Here's how the part is built. I have some questions about the finished solid (model axes, mm). A direction names the side the tool comes from. Coordinates: 2 decimals unless noted, no trailing zeros. Write each loop counter-clockwise with the first axis right and the second up, starting at its lowest first coordinate (ties: lowest second). Pieces come first, ordered by that corner, then holes. Notation, with made-up numbers: (34.5, 66.25) -> (54.5, 66.25) arc R23 ccw to (54.5, 98.25) -> close; hole circle Ø7 at (54, -7). An arc over 180 degrees is marked (long way). Answer in a Markdown table with one row per item. Add a question column.
from build123d import *

# Parameters (mm, degrees)
SKETCH2_R           = 19.05
SKETCH2_R_2         = 6.688770164
SKETCH2_R_3         = 2.328803663
BOSS_EXTRUDE1_DEPTH = 6.35
SKETCH3_R           = 10.424468921
BOSS_EXTRUDE2_DEPTH = 11.176
FILLET1_R           = 2.54


with BuildPart() as part:
    # Sketch2 → Boss-Extrude1 (new body)
    with BuildSketch(Plane(origin=(0, 0, 0), x_dir=(1, 0, 0), z_dir=(0, 1, 0))):
        with Locations(Location((0, 0, 0), (0, 0, 270))):
            Circle(SKETCH2_R)
        with Locations(Location((0, 0, 0), (0, 0, 270))):
            Circle(SKETCH2_R_2, mode=Mode.SUBTRACT)
        with Locations(Location((0, 13.4441798, 0), (0, 0, 270))):
            Circle(SKETCH2_R_3, mode=Mode.SUBTRACT)
        with Locations(Location((13.4441798, 0, 0), (0, 0, 270))):
            Circle(SKETCH2_R_3, mode=Mode.SUBTRACT)
        with Locations(Location((0, -13.4441798, 0), (0, 0, 270))):
            Circle(SKETCH2_R_3, mode=Mode.SUBTRACT)
        with Locations(Location((-13.4441798, 0, 0), (0, 0, 270))):
            Circle(SKETCH2_R_3, mode=Mode.SUBTRACT)
    extrude(amount=BOSS_EXTRUDE1_DEPTH)

    # Sketch3 → Boss-Extrude2 (add)
    with BuildSketch(Plane(origin=(0, 6.35, 0), x_dir=(1, 0, 0), z_dir=(0, 1, 0))):
        with Locations(Location((0, 0, 0), (0, 0, 270))):
            Circle(SKETCH3_R)
    extrude(amount=BOSS_EXTRUDE2_DEPTH)

    # Fillet1
    fillet1_edges = [part.edges().sort_by_distance(p)[0] for p in [
        (0, 17.526, -10.424468921),
    ]]
    fillet(fillet1_edges, radius=FILLET1_R)


with BuildPart() as body_2:
    # Sketch5 → Revolve1 (revolve)
    with BuildSketch(Plane(origin=(0, 17.526, 0), x_dir=(1, 0, 0), z_dir=(0, 1, 0))):
        with BuildLine():
            Line((0, 7.884468921), (0, -7.884468921))
            ThreePointArc((0, -7.884468921), (7.884468921, 0), (0, 7.884468921))
        make_face()
    revolve(axis=Axis((0, 17.526, -14.295685005), (0, 0, 1)))


with BuildPart() as part_1:
    add(part.part)

    # Combine1: cut body 2
    add(body_2.part, mode=Mode.SUBTRACT)


solid = part_1.part
Q1. If we mould it in two halves opening along X, with no side actions, what happens to faces 1 (the cylindrical face through (0.7, 3.131, -11.223)), 2 (the flat face through (0, 0, 8)), 3 (the cylindrical face through (3.131, 10.608, 9.943))? For each: pulls with the +X half, pulls with the -X half, needs draft (parallel to the pull), parting line crosses it, or undercut.
Q2. I'm going to push flat-ended pins straight in: P1, Ø3, axis at y = 4.5, z = 14, coming from the -X side; P2, Ø3, axis at x = -14.5, z = -6.5, coming from the +Y side; P3, Ø8, axis at x = 0.5, z = -12.5, coming from the -Y side; P4, Ø3.5, axis at x = -13.44, z = 0, coming from the +Y side (3 decimals). Where does each tip first touch, or does it pass through?
Q3. Imagine slicing it at A-A on x = 0. Please give me the cut outline in (y, z).
Q4. Imagine slicing it at B-B on z = 0. Please give me the cut outline in (x, y).
Q5. Imagine slicing it at D-D on x = 12.5. Please give me the cut outline in (y, z).
Q6. Imagine slicing it at C-C on z = 12.5. Please give me the cut outline in (x, y), plus the area to 3 significant figures.
Q7. I need wall thicknesses on line 1 (X direction, y = 3.75, z = 0); line 2 (Y direction, x = -3.5, z = 17); line 3 (Z direction, x = -1, y = 6). Which ranges of each line are inside material? Lowest first, please. Write a range as [from, to].
Q8. For faces 4 (the flat face through (-8, 6.35, 8)), 5 (the cylindrical face through (15.41, 3.13, 1.25)), 6 (the flat face through (0, 6.35, 0)), which set-ups out of +Z, -Z, +X, -X, +Y, -Y let a thin tool reach every point of the face, with its end or its side?
Result sheet:
| question | item | result |
|---|---|---|
| 1 | face 1 | undercut |
| 1 | face 2 | needs draft |
| 1 | face 3 | parting line crosses it |
| 2 | P1 | stops at x = -14.38 |
| 2 | P2 | stops at y = 6.35 |
| 2 | P3 | stops at y = 0 |
| 2 | P4 | passes through |
| 3 | outline | (0, -19.05) -> (6.35, -19.05) -> (6.35, -15.77) -> (0, -15.77) -> close; (0, -11.12) -> (6.35, -11.12) -> (6.35, -10.42) -> (14.99, -10.42) arc R2.54 ccw to (17.53, -7.88) arc R7.88 cw to (17.53, 7.88) arc R2.54 ccw to (14.99, 10.42) -> (6.35, 10.42) -> (6.35, 11.12) -> (0, 11.12) -> (0, 6.69) -> (6.35, 6.69) -> (6.35, -6.69) -> (0, -6.69) -> close; (0, 15.77) -> (6.35, 15.77) -> (6.35, 19.05) -> (0, 19.05) -> close |
| 4 | outline | (-19.05, 0) -> (-15.77, 0) -> (-15.77, 6.35) -> (-19.05, 6.35) -> close; (-11.12, 0) -> (-6.69, 0) -> (-6.69, 6.35) -> (6.69, 6.35) -> (6.69, 0) -> (11.12, 0) -> (11.12, 6.35) -> (10.42, 6.35) -> (10.42, 14.99) arc R2.54 ccw to (7.88, 17.53) arc R7.88 cw to (-7.88, 17.53) arc R2.54 ccw to (-10.42, 14.99) -> (-10.42, 6.35) -> (-11.12, 6.35) -> close; (15.77, 0) -> (19.05, 0) -> (19.05, 6.35) -> (15.77, 6.35) -> close |
| 5 | outline | (0, -14.38) -> (6.35, -14.38) -> (6.35, -2.13) -> (0, -2.13) -> close; (0, 2.13) -> (6.35, 2.13) -> (6.35, 14.38) -> (0, 14.38) -> close |
| 6 | outline | (-14.38, 0) -> (-2.13, 0) -> (-2.13, 6.35) -> (-14.38, 6.35) -> close; (2.13, 0) -> (14.38, 0) -> (14.38, 6.35) -> (2.13, 6.35) -> close |
| 6 | area | 156 mm^2 |
| 7 | line 1 | x = [-19.05, -15.77], [-11.12, -6.69], [6.69, 11.12], [15.77, 19.05] |
| 7 | line 2 | y = [0, 6.35] |
| 7 | line 3 | z = [-19.02, -15.55], [-11.34, -6.61], [6.61, 11.34], [15.55, 19.02] |
| 8 | face 4 | +Y |
| 8 | face 5 | +Y, -Y |
| 8 | face 6 | -Y |
